Build history of the part. All positions in model axes, mm. A direction names the side the tool comes from. Give positions to 0.01 mm unless a question says otherwise; leave off trailing zeros. Loops run counter-clockwise (first coordinate to the right, second up) from the corner with the lowest first, then second, coordinate; pieces in that order, holes last.
1) Band-saw the part on B-B on y = 8.4. List the corners of the cut face in (x, z) (3 decimals), then the cut area to 3 significant figures.
2) Two-plate mould, pull along Y, no slides. Class faces 1 (the flat face through (0.986, 13.861, 0.71)), 2 (the flat face through (60, 16, 0)), 3 (the cylindrical face through (120.84, 17.37, 5.1)): +Y half, -Y half, draft (parallel to the pull), parting line (faces both ways), or undercut.
3) Flat gauge pins, fed straight in: P1, Ø4, axis at y = 12, z = 5.5, coming from the -X side; P2, Ø1.1, axis at x = 43, z = 1, coming from the +Y side; P3, Ø0.5, axis at x = 121, z = 11, coming from the -Y side. Where does each tip first touch, or does it go through?
4) Band-saw the part on C-C on x = 105.5. List the corners of the cut face in (y, z).
5) 3-axis set-ups, long thin cutter, end or side, ignore diameter. For faces 4 (the cylindrical face through (76.709, 13.337, 0.69)), 5 (the flat face through (120.5, 2.66, 6.1)), 6 (the flat face through (9.85, 1.89, 0.69)), 7 (the cylindrical face through (120.84, 14.14, 5.07)), 8 (the flat face through (59, 16, 1.4)): which of +Z, -Z, +X, -X, +Y, -Y reach the whole face in a straight line?
6) Band-saw the part on D-D on y = 19.75. List the corners of the cut face in (x, z).
7) Wall check: line 1 (X direction, y = 8.4, z = 0.4) (3 decimals); line 2 (Z direction, x = 43, y = 4.5); line 3 (X direction, y = 4, z = 8.5). Give the ranges that are in metal, low to high.
8) Band-saw the part on A-A on z = 9. List the corners of the cut face in (x, y), then the cut area to 3 significant figures.
Autodesk Fusion 360 part; units mm, degrees
sketch "스케치1" plane through (0, 0, 0) normal (0, 0, 1) x (1, 0, 0)
  line L0 (11.75, 18.6) -> (114.5, 18.6)
  line L1 (114.5, 18.6) -> (114.5, 0)
  line L2 (114.5, 0) -> (11.75, 0)
  line L3 (11.75, 0) -> (11.75, 18.6)
  line L4 (0, 14.875) -> (8, 14.875)
  line L5 (8, 14.875) -> (8, 3.725)
  line L6 (8, 3.725) -> (0, 3.725)
  line L7 (0, 3.725) -> (0, 14.875)
  line L8 (0, 9.3) -> (8, 9.3) construction
  line L9 (8, 14.875) -> (11.75, 18.6)
  line L10 (8, 3.725) -> (11.75, 0)
  line L11 (1.75, 0) -> (22.5, 0)
  line L12 (0, 1.75) -> (0, 22.5)
  line L13 (120, 21.36) -> (117.25, 21.36)
  line L14 (117.25, 21.36) -> (117.25, 2.66)
  line L15 (117.25, 2.66) -> (120, 2.66)
  line L16 (120, 2.66) -> (120, 21.36)
  line L17 (114.5, 0) -> (144, 0) construction
  line L18 (114.5, 18.6) -> (117.25, 21.36)
  line L19 (114.5, 0) -> (117.25, 2.66)
  line L20 (120, 21.36) -> (121.7, 21.36)
  line L21 (121.7, 21.36) -> (121.7, 2.66)
  line L22 (121.7, 2.66) -> (120, 2.66)
  line L23 (120, 2.66) -> (120, 21.36)
  dimension "d1" = 102.75
  dimension "d2" = 18.6
  dimension "d3" = 8
  dimension "d4" = 11.15
  dimension "d5" = 3.75
  dimension "d6" = 18.7
  dimension "d7" = 2.66
  dimension "d8" = 2.75
  dimension "d9" = 2.75
  dimension "d10" = 1.7
extrude "돌출1" add sketch "스케치1" along normal blind 1.4 contours L0 L1 L2 L3 L11 | L3 L5 L9 L10 | L1 L14 L18 L19 | L4 L5 L6 L7 L12 | L13 L14 L15 L16 L23
extrude "돌출2" add sketch "스케치1" along normal blind 12.4 contours L16 L20 L21 L22 L23
chamfer "모따기1" distance 2 angle 45 2 edges at (0, 3.725, 0.7) (0, 14.875, 0.7)
sketch "스케치2" plane through (121.7, 0, 0) normal (1, 0, 0) x (0, 1, 0)
  line L0 (2.66, 0) -> (21.36, 0)
  line L1 (21.36, 0) -> (21.36, 12.4)
  line L2 (21.36, 12.4) -> (2.66, 12.4)
  line L3 (2.66, 12.4) -> (2.66, 0)
  line L4 (13.54, 12.4) -> (17.94, 12.4)
  line L5 (17.94, 12.4) -> (17.94, 4.5)
  line L6 (17.94, 4.5) -> (13.54, 4.5)
  line L7 (13.54, 4.5) -> (13.54, 12.4)
  dimension "d16" = 3.42
  dimension "d17" = 4.4
  dimension "d18" = 7.9
extrude "돌출3" cut sketch "스케치2" against normal blind 3 contours L2 L4 L5 L6 L7
fillet "모깎기1" radius 2 2 edges at (120.85, 13.54, 4.5) (120.85, 17.94, 4.5)
sketch "스케치3" plane through (0, 0, 1.4) normal (0, 0, 1) x (-1, 0, 0)
  line L0 (-2, -14.875) -> (0, -12.875)
  line L1 (0, -12.875) -> (0, -5.725)
  line L2 (0, -5.725) -> (-2, -3.725)
  line L3 (-2, -3.725) -> (-8, -3.725)
  line L4 (-8, -3.725) -> (-11.75, 0)
  line L5 (-11.75, 0) -> (-114.5, 0)
  line L6 (-114.5, 0) -> (-117.25, -2.66)
  line L7 (-117.25, -2.66) -> (-120, -2.66)
  line L8 (-120, -2.66) -> (-120, -21.36)
  line L9 (-120, -21.36) -> (-117.25, -21.36)
  line L10 (-117.25, -21.36) -> (-114.5, -18.6)
  line L11 (-114.5, -18.6) -> (-11.75, -18.6)
  line L12 (-11.75, -18.6) -> (-8, -14.875)
  line L13 (-8, -14.875) -> (-2, -14.875)
  line L14 (7.5, -3.3) -> (-137.5, -3.3) construction
  line L15 (-114.5, 0) -> (-11.75, 0)
  line L16 (7.5, -14) -> (-137.5, -14) construction
  line L17 (-57, -14) -> (-77.5, -14)
  line L18 (-58.4, -3.3) -> (-76.1, -3.3)
  line L19 (-57, -14) -> (-58.4, -3.3)
  line L20 (-77.5, -14) -> (-76.1, -3.3)
  line L21 (-67.25, -32) -> (-67.25, 14) construction
  line L22 (-57, -26) -> (-57, 12) construction
  line L23 (-77.5, -26) -> (-77.5, 12) construction
  circle A0 centre (-54.495, -8.4) radius 1.8
  circle A1 centre (-79.705, -8.4) radius 1.8
  line L24 (-77.905, -12) -> (-77.905, -5.5195) construction
  line L25 (-56.295, -12) -> (-56.295, -5.5195) construction
  line L26 (-53, -6.6) -> (-81.5, -6.6) construction
  dimension "d23" = 3.3
  dimension "d24" = 10.7
  dimension "d25" = 20.5
  dimension "d26" = 17.7
  dimension "d27" = 42.5
  dimension "d28" = 3.6
  dimension "d30" = 0.705
  dimension "d31" = 0.405
  dimension "d32" = 3.3
extrude "돌출4" cut sketch "스케치3" against normal blind 2 contours L17 L18 L19 L20 | A0 | A1
fillet "모깎기2" radius 2 4 edges at (77.5, 14, 0.7) (57, 14, 0.7) (76.1, 3.3, 0.7) (58.4, 3.3, 0.7)
Findings below:
1. outline: (0, 0) - (52.695, 0) - (52.695, 1.4) - (0, 1.4) - close; (56.295, 0) - (57.733, 0) - (57.733, 1.4) - (56.295, 1.4) - close; (76.767, 0) - (77.905, 0) - (77.905, 1.4) - (76.767, 1.4) - close; (81.505, 0) - (121.7, 0) - (121.7, 12.4) - (120, 12.4) - (120, 1.4) - (81.505, 1.4) - close
1. area: 152 mm2
2. face 1: +Y half
2. face 2: draft
2. face 3: undercut
3. P1: stops at x = 120
3. P2: stops at y = 18.6
3. P3: stops at y = 2.66
4. outline: (0, 0) - (18.6, 0) - (18.6, 1.4) - (0, 1.4) - close
5. face 4: +Z, -Z
5. face 5: +Z, -Z, +X, -Y
5. face 6: +Z, -Z, -X, -Y
5. face 7: +Z, +X, -X
5. face 8: +Z, -X, +Y, -Y
6. outline: (115.65, 0) - (121.7, 0) - (121.7, 12.4) - (120, 12.4) - (120, 1.4) - (115.65, 1.4) - close
7. line 1: x = 0 to 52.695, 56.295 to 57.733, 76.767 to 77.905, 81.505 to 121.7
7. line 2: z = 0 to 1.4
7. line 3: x = 120 to 121.7
8. outline: (120, 2.66) - (121.7, 2.66) - (121.7, 13.54) - (120, 13.54) - close; (120, 17.94) - (121.7, 17.94) - (121.7, 21.36) - (120, 21.36) - close
8. area: 24.3 mm2
